from build123d import *

# Parameters (mm, degrees)
SKETCH1_W               = 880
SKETCH1_H               = 580
BOSS_EXTRUDE1_DEPTH     = 100
SKETCH2_W               = 160
SKETCH2_H               = 580
CUT_EXTRUDE1_DEPTH      = 30
SKETCH3_W               = 210
SKETCH3_H               = 580
CUT_EXTRUDE2_DEPTH      = 30
SKETCH4_R               = 37
CUT_EXTRUDE3_DEPTH      = 264
SKETCH6_R               = 30
CUT_EXTRUDE5_DEPTH      = 271
SKETCH7_R               = 35
CUT_EXTRUDE6_DEPTH      = 10
SKETCH9_R               = 4
CUT_EXTRUDE14_DEPTH     = 500
CIRPATTERN2_COUNT       = 4
MIRROR2_COPY_1_SKETCH_R = 4
MIRROR2_COPY_1_DEPTH    = 500
MIRROR2_COPY_2_SKETCH_R = 4
MIRROR2_COPY_2_DEPTH    = 500
MIRROR2_COPY_3_SKETCH_R = 4
MIRROR2_COPY_3_DEPTH    = 500


with BuildPart() as part:
    # Sketch1 → Boss-Extrude1 (new body)
    with BuildSketch(Plane(origin=(0, 0, 0), x_dir=(1, 0, 0), z_dir=(0, 1, 0))):
        Rectangle(SKETCH1_W, SKETCH1_H)
    extrude(amount=BOSS_EXTRUDE1_DEPTH)

    # Sketch2 → Cut-Extrude1 (cut)
    with BuildSketch(Plane(origin=(0, 100, 0), x_dir=(1, 0, 0), z_dir=(0, 1, 0))):
        with Locations((-145, 0)):
            Rectangle(SKETCH2_W, SKETCH2_H)
        with Locations((145, 0)):
            Rectangle(SKETCH2_W, SKETCH2_H)
    extrude(amount=-CUT_EXTRUDE1_DEPTH, mode=Mode.SUBTRACT)

    # Sketch3 → Cut-Extrude2 (cut)
    with BuildSketch(Plane(origin=(0, 100, 0), x_dir=(1, 0, 0), z_dir=(0, 1, 0))):
        with Locations((170, 0)):
            Rectangle(SKETCH3_W, SKETCH3_H)
        with Locations((-170, 0)):
            Rectangle(SKETCH3_W, SKETCH3_H)
    extrude(amount=-CUT_EXTRUDE2_DEPTH, mode=Mode.SUBTRACT)

    # Sketch4 → Cut-Extrude3 (cut)
    with BuildSketch(Plane(origin=(0, 70, 0), x_dir=(1, 0, 0), z_dir=(0, 1, 0))):
        with Locations(Location((-159, 0, 0), (0, 0, 270))):
            Circle(SKETCH4_R)
        with Locations(Location((159, 0, 0), (0, 0, 270))):
            Circle(SKETCH4_R)
    extrude(amount=-CUT_EXTRUDE3_DEPTH, mode=Mode.SUBTRACT)

    # Sketch6 → Cut-Extrude5 (cut)
    with BuildSketch(Plane(origin=(0, 100, 0), x_dir=(1, 0, 0), z_dir=(0, 1, 0))):
        with Locations(Location((-340, 200, 0), (0, 0, 270))):
            Circle(SKETCH6_R)
        with Locations(Location((340, 200, 0), (0, 0, 270))):
            Circle(SKETCH6_R)
        with Locations(Location((340, -200, 0), (0, 0, 270))):
            Circle(SKETCH6_R)
        with Locations(Location((-340, -200, 0), (0, 0, 270))):
            Circle(SKETCH6_R)
    extrude(amount=-CUT_EXTRUDE5_DEPTH, mode=Mode.SUBTRACT)

    # Sketch7 → Cut-Extrude6 (cut)
    with BuildSketch(Plane.XZ):
        with Locations(Location((-340, 200, 0), (0, 0, 270))):
            Circle(SKETCH7_R)
        with Locations(Location((340, 200, 0), (0, 0, 270))):
            Circle(SKETCH7_R)
        with Locations(Location((-340, -200, 0), (0, 0, 270))):
            Circle(SKETCH7_R)
        with Locations(Location((340, -200, 0), (0, 0, 270))):
            Circle(SKETCH7_R)
    extrude(amount=-CUT_EXTRUDE6_DEPTH, mode=Mode.SUBTRACT)

    # Sketch9 → Cut-Extrude14 (cut)
    with BuildSketch(Plane.XZ):
        with Locations(Location((-129.655068581, 29.344931419, 0), (0, 0, 270))):
            Circle(SKETCH9_R)
    cut_extrude14 = extrude(amount=-CUT_EXTRUDE14_DEPTH, mode=Mode.SUBTRACT)

    # CirPattern2: Cut-Extrude14 ×4 about axis
    cirpattern2_axis = Axis((-159, 0, 0), (0, 1, 0))
    for i in range(1, CIRPATTERN2_COUNT):
        add(cut_extrude14.rotate(cirpattern2_axis, i * 360 / CIRPATTERN2_COUNT), mode=Mode.SUBTRACT)

    # Mirror2: Cut-Extrude14 across plane
    add(cut_extrude14.mirror(Plane(origin=(0, 0, 0), x_dir=(0, 0, 1), z_dir=(1, 0, 0))), mode=Mode.SUBTRACT)

    # Mirror2 copy 1 sketch → Mirror2 copy 1 (cut)
    with BuildSketch(Plane(origin=(159, 0, -159), x_dir=(0, 0, -1), z_dir=(0, -1, 0))):
        with Locations((-129.655068581, -29.344931419)):
            Circle(MIRROR2_COPY_1_SKETCH_R)
    extrude(amount=-MIRROR2_COPY_1_DEPTH, mode=Mode.SUBTRACT)

    # Mirror2 copy 2 sketch → Mirror2 copy 2 (cut)
    with BuildSketch(Plane(origin=(318, 0, 0), x_dir=(1, 0, 0), z_dir=(0, -1, 0))):
        with Locations((-129.655068581, -29.344931419)):
            Circle(MIRROR2_COPY_2_SKETCH_R)
    extrude(amount=-MIRROR2_COPY_2_DEPTH, mode=Mode.SUBTRACT)

    # Mirror2 copy 3 sketch → Mirror2 copy 3 (cut)
    with BuildSketch(Plane(origin=(159, 0, 159), x_dir=(0, 0, 1), z_dir=(0, -1, 0))):
        with Locations((-129.655068581, -29.344931419)):
            Circle(MIRROR2_COPY_3_SKETCH_R)
    extrude(amount=-MIRROR2_COPY_3_DEPTH, mode=Mode.SUBTRACT)


solid = part.part
Geometry check sheet. Reference: the model listing, model coordinates, mm. A direction names the side the tool comes from. Give positions to 0.01 mm unless a question says otherwise; leave off trailing zeros. Write each loop counter-clockwise with the first axis right and the second up, starting at its lowest first coordinate (ties: lowest second). Pieces come first, ordered by that corner, then holes.
1) Cross-section at C-C (z = -207). Record the boundary of the cut face in (x, y).
Values follow:
outline: (-440, 0) - (-374.29, 0) - (-374.29, 10) - (-369.17, 10) - (-369.17, 100) - (-440, 100) - close; (-310.83, 10) - (-305.71, 10) - (-305.71, 0) - (305.71, 0) - (305.71, 10) - (310.83, 10) - (310.83, 100) - (275, 100) - (275, 70) - (65, 70) - (65, 100) - (-65, 100) - (-65, 70) - (-275, 70) - (-275, 100) - (-310.83, 100) - close; (369.17, 10) - (374.29, 10) - (374.29, 0) - (440, 0) - (440, 100) - (369.17, 100) - close
2) Cross-section at D-D (y = 41). Count the separate pieces of the cut face and the enclosed holes in it, plus the area to 3 significant figures.
Values follow:
separate pieces: 1
enclosed holes: 14
area: 490,000 mm2
3) Cross-section at B-B (x = 159). Record the boundary of the cut face in (y, z).
Values follow:
outline: (0, -290) - (70, -290) - (70, -37) - (0, -37) - close; (0, 37) - (70, 37) - (70, 290) - (0, 290) - close
4) Go/stop test with flat-tipped pins: pin 1 Ø7 at (x, z) = (129.66, -29.34) entering from +Y; pin 2 Ø12 at (x, z) = (-269.5, 138) entering from -Y. Record where each tip stops, or that it passes through.
Values follow:
pin 1: passes through
pin 2: stops at y = 0
5) Cross-section at A-A (x = 340). Record the boundary of the cut face in (y, z), plus the area to 3 significant figures.
Values follow:
outline: (0, -290) - (100, -290) - (100, -230) - (10, -230) - (10, -235) - (0, -235) - close; (0, -165) - (10, -165) - (10, -170) - (100, -170) - (100, 170) - (10, 170) - (10, 165) - (0, 165) - close; (0, 235) - (10, 235) - (10, 230) - (100, 230) - (100, 290) - (0, 290) - close
area: 45,800 mm2
6) Release check for a two-part mould opening along Z. For faces 4 (the face through (-6, 38, 290)), 5 (the face through (-6, 0, -4)), 6 (the face through (-366.615, 55.63, 213.843)) record: released by +Z, released by -Z, zero draft, split by the parting line, or undercut.
Values follow:
face 4: released by +Z
face 5: zero draft
face 6: undercut
7) Set-up check for faces 1 (the face through (356, 10, -226)), 2 (the face through (313.385, 55.63, 213.843)), 3 (the face through (-65, 85, 4)): record each of +Z, -Z, +X, -X, +Y, -Y from which the full face is reachable in a straight line by a thin tool's end or side.
Values follow:
face 1: -Y
face 2: +Y, -Y
face 3: +Z, -Z, +Y
8) Thickness scan on line 1 (X direction, y = 18, z = 0); line 2 (X direction, y = 96.5, z = -27.5); line 3 (X direction, y = 83, z = 202.5). Record the ranges inside material, lowest first.
Values follow:
line 1: x = -440 to -196, -122 to 122, 196 to 440
line 2: x = -440 to -275, -65 to 65, 275 to 440
line 3: x = -440 to -369.9, -310.1 to -275, -65 to 65, 275 to 310.1, 369.9 to 440
